```python
from build123d import *

# Parameters (mm, degrees)
EXTRUSION1_DEPTH = 20
ESQUISSE2_R      = 1.5
EXTRUSION2_DEPTH = 20
ESQUISSE3_R      = 1.5
EXTRUSION3_DEPTH = 10


with BuildPart() as part:
    # Esquisse1 → Extrusion1 (new body)
    with BuildSketch(Plane.XY):
        Polygon((-18.714271359, 3.498089172), (-18.714271359, -16.501910828), (1.285728641, -16.501910828), (1.285728641, -15.001910828), (-17.214271359, -15.001910828), (-17.214271359, 3.498089172), align=None)
    extrude(amount=EXTRUSION1_DEPTH)

    # Esquisse2 → Extrusion2 (cut)
    with BuildSketch(Plane(origin=(0, -15.001910828, 0), x_dir=(-1, 0, 0), z_dir=(0, 1, 0))):
        with Locations((8.633652734, 14)):
            Circle(ESQUISSE2_R)
        with Locations((8.633652734, 6)):
            Circle(ESQUISSE2_R)
    extrude(amount=-EXTRUSION2_DEPTH, mode=Mode.SUBTRACT)

    # Esquisse3 → Extrusion3 (cut)
    with BuildSketch(Plane.ZY.offset(18.714271359)):
        with Locations(Location((10, -10.501910828, 0), (0, 0, 270))):
            Circle(ESQUISSE3_R)
        with Locations(Location((10, -2.501910828, 0), (0, 0, 270))):
            Circle(ESQUISSE3_R)
    extrude(amount=-EXTRUSION3_DEPTH, mode=Mode.SUBTRACT)


solid = part.part
```
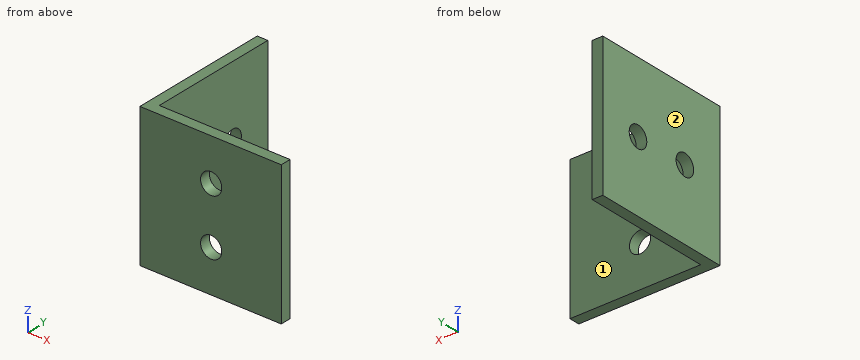
Geometry: final body of the model. Coordinates: model frame, mm. Face numbers are marked on the shaded views. A direction names the side the tool comes from. Coordinates: 2 decimals unless noted, no trailing zeros. Order: outer loops, then holes, each group sorted by start corner. A loop starts at its lowest first (then second) coordinate and runs counter-clockwise, first axis right, second up. Notation, with made-up numbers: (19.25, -27.75) -> (70.25, -27.75) arc R5 ccw to (70.25, -22.75) -> close; hole circle Ø9 at (61.5, 83). An arc over 180 degrees is marked (long way). Write each question's results on one line, items separated by ' | '. Start each with the question number.
1) Material intervals for line 1 along Y through (x, z) = (-16.75, 13.25); line 2 along X through (y, z) = (-5.25, 5), sorted ascending.
2) Set-up query: the marked faces 1 and 2. Return all of +Z, -Z, +X, -X, +Y, -Y with unobstructed straight access to the full face (end or side cutting, diameter ignored); none if empty.
3) First-contact query: pin 1 (6 mm diameter, centred on y = -4, z = 18, fed in from +X); pin 2 (2.5 mm diameter, centred on y = -2.5, z = 10, fed in from -X); pin 3 (4 mm diameter, centred on x = -8.63, z = 14, fed in from +Y). Flat tips, straight axial feed; report the tip coordinate or a pass-through.
4) Cut plane B-B, the plane z = 10. Output: boundary loops of the cut face in (x, y).
5) Cut plane C-C, the plane y = -11.5. Output: boundary loops of the cut face in (x, z), and give its area (3 significant figures).
6) Cut plane A-A, the plane z = 6. Output: boundary loops of the cut face in (x, y).
7) Cut plane D-D, the plane x = -10.5. Output: boundary loops of the cut face in (y, z), and give its area (3 significant figures).
Checks:
1) line 1: -16.5 to -15 | line 2: -18.71 to -17.21
2) face 1: +Z, -Z, +X, +Y | face 2: +Z, -Z, -X, +Y, -Y
3) pin 1: x = -17.21 | pin 2: through | pin 3: y = -15
4) outline: (-18.71, -16.5) -> (1.29, -16.5) -> (1.29, -15) -> (-17.21, -15) -> (-17.21, -12) -> (-18.71, -12) -> close; (-18.71, -9) -> (-17.21, -9) -> (-17.21, -4) -> (-18.71, -4) -> close; (-18.71, -1) -> (-17.21, -1) -> (-17.21, 3.5) -> (-18.71, 3.5) -> close
5) outline: (-18.71, 0) -> (-17.21, 0) -> (-17.21, 8.88) -> (-18.71, 8.88) -> close; (-18.71, 11.12) -> (-17.21, 11.12) -> (-17.21, 20) -> (-18.71, 20) -> close | area: 26.6 mm^2
6) outline: (-18.71, -16.5) -> (-10.13, -16.5) -> (-10.13, -15) -> (-17.21, -15) -> (-17.21, 3.5) -> (-18.71, 3.5) -> close; (-7.13, -16.5) -> (1.29, -16.5) -> (1.29, -15) -> (-7.13, -15) -> close
7) outline: (-16.5, 0) -> (-15, 0) -> (-15, 20) -> (-16.5, 20) -> close | area: 30.0 mm^2
